```python
from build123d import *

# Parameters (mm, degrees)
F0_R     = 3.95
F1_DEPTH = 6


with BuildPart() as f1:
    # F0 (on Top) → F1 (new body)
    with BuildSketch(Plane.XY):
        Polygon((53.84666, 30.722071), (-76.15334, 30.722071), (-76.15334, 4.438029), (23.84666, -43.277929), (53.84666, -43.277929), (53.84666, -35.277929), (40.64666, -35.277929), (40.64666, -16.499616), (34.84666, 4.722071), (48.84666, 4.722071), (48.84666, -9.277929), (53.84666, -9.277929), align=None)
        Polygon((29.634969, -12.120992), (20.942271, -27.102214), (3.621804, -27.064728), (-5.005966, -12.04602), (3.686731, 2.935202), (21.007199, 2.897716), align=None, mode=Mode.SUBTRACT)
        Polygon((-5.652112, 7.919449), (-12.925933, -4.547502), (-27.359539, -4.481664), (-34.519325, 8.051125), (-27.245504, 20.518076), (-12.811898, 20.452238), align=None, mode=Mode.SUBTRACT)
        Polygon((-41.32622, 15.791604), (-45.621206, 8.456361), (-54.121206, 8.508307), (-58.32622, 15.895495), (-54.031233, 23.230739), (-45.531233, 23.178793), align=None, mode=Mode.SUBTRACT)
        with Locations((-69.15334, 23.722071)):
            Circle(F0_R, mode=Mode.SUBTRACT)
        Polygon((7.283409, 17.353729), (12.993321, 27.390174), (24.540094, 27.463468), (30.376955, 17.500317), (24.667043, 7.463871), (13.12027, 7.390577), align=None, mode=Mode.SUBTRACT)
        with Locations((46.84666, 23.722071)):
            Circle(F0_R, mode=Mode.SUBTRACT)
    extrude(amount=F1_DEPTH)


solid = f1.part
```
Design review of the part built by this model. Coordinates are the model's own, in mm. A direction names the side the tool comes from. Give positions to 0.01 mm unless a question says otherwise; leave off trailing zeros. Order: outer loops, then holes, each group sorted by start corner. A loop starts at its lowest first (then second) coordinate and runs counter-clockwise, first axis right, second up. Notation, with made-up numbers: M -35,0.25 L -17,0.25 A10 ccw -17,6.25 Z; hole C 73.25,24.25 d2. An arc over 180 degrees is marked long. One line per question, with ' | ' between items. Start each with the question number.
Q1. The part is to be moulded in two halves that separate along X. For faces 4 (the face through (-56.194, 12.15, 2.958)), 5 (the face through (-26.853, -19.086, 2.958)), 6 (the face through (-43.44, 12.18, 2.96)), 7 (the face through (53.847, -39, 3)), say which applies: +X half, -X half, draft (parallel to the pull), parting line (faces both ways), or undercut.
Q2. Machinability: for faces 1 (the face through (-12, -6, 6)), 2 (the face through (-9.24, 1.77, 2.96)), 3 (the face through (47, -35.278, 3)), which of the approach directions +Z, -Z, +X, -X, +Y, -Y give a long, thin tool a straight path to every point of the face, cutting with its end or side? Answer none if there is none.
Q3. We need section B-B (y = -22). Write out the cut boundary in (x, z).
Q4. We need section D-D (z = 4.3). State how many separate pieces and enclosed holes the cut face has, plus the area to 3 significant figures.
Q5. For L1, parallel to Y at x = 46.5, z = 2.35; L2, parallel to X at y = -5.5, z = 2.25; L3, parallel to X at y = -0.5, z = 2.3, list the stretches that pass through material, from the lowest coordinate up. Write a range as [from, to].
Q6. We need section C-C (x = -50). Write out the cut boundary in (y, z).
Q7. We need section A-A (x = 28). Write out the cut boundary in (y, z).
Q8. For pin 1 Ø9 at (x, y) = (46.85, 23.72) entering from +Z; pin 2 Ø3 at (y, z) = (-27, 4.5) entering from +X; pin 3 Ø3 at (y, z) = (0, 2.5) entering from -X; pin 4 Ø1 at (y, z) = (-13, 2) entering from -X, all flat-tipped, find the tip position at first contact; note any pin that passes through.
Returned:
1) face 4: undercut | face 5: -X half | face 6: undercut | face 7: +X half
2) face 1: +Z, +X, -X, +Y, -Y | face 2: +Z, -Z | face 3: +Z, -Z, +X
3) outline: M -20.75,0 L 0.71,0 L 0.71,6 L -20.75,6 Z; M 23.9,0 L 40.65,0 L 40.65,6 L 23.9,6 Z
4) separate pieces: 1 | enclosed holes: 6 | area: 4,760 mm2
5) L1: [-43.28, -35.28], [4.72, 19.79], [27.66, 30.72] | L2: [-55.33, -1.21], [25.83, 37.64], [48.85, 53.85] | L3: [-65.8, -29.63], [-10.56, 1.69], [22.96, 36.27], [48.85, 53.85]
6) outline: M -8.04,0 L 8.48,0 L 8.48,6 L -8.04,6 Z; M 23.21,0 L 30.72,0 L 30.72,6 L 23.21,6 Z
7) outline: M -43.28,0 L -14.94,0 L -14.94,6 L -43.28,6 Z; M -9.27,0 L 13.32,0 L 13.32,6 L -9.27,6 Z; M 21.56,0 L 30.72,0 L 30.72,6 L 21.56,6 Z
8) pin 1: z = 6 | pin 2: x = 40.65 | pin 3: x = -70 | pin 4: x = -40.66
